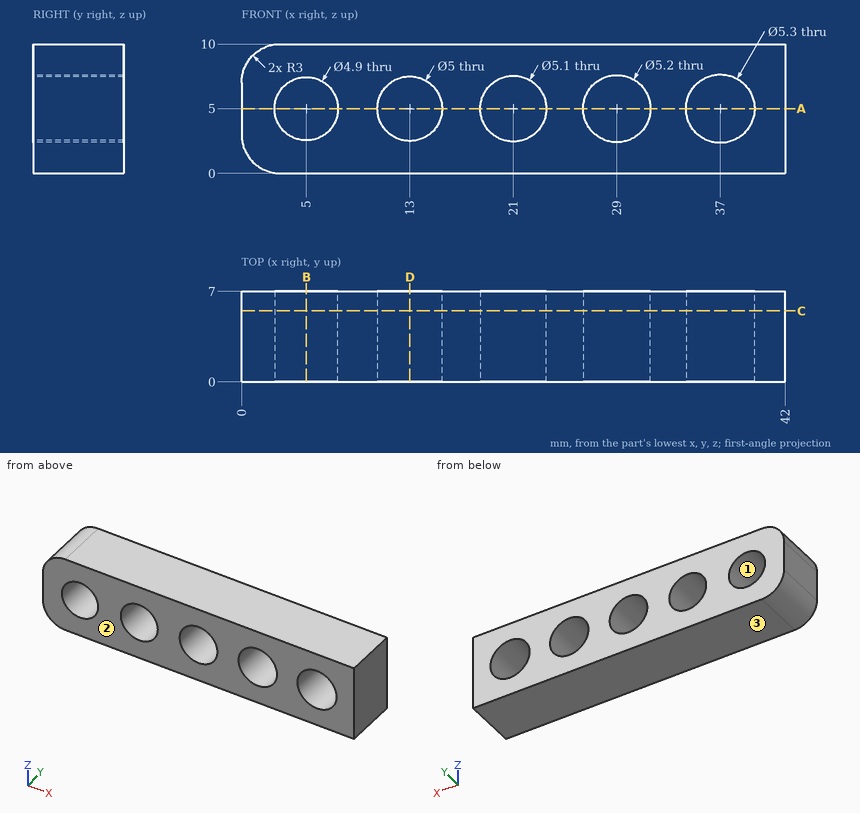
The figure shows three views and two pictorial views of one solid part (mm, origin at its lowest corner). Answer the questions. Round coordinates to 2 decimals unless told otherwise and drop trailing zeros. Order: outer loops, then holes, each group sorted by start corner. A loop starts at its lowest first (then second) coordinate and runs counter-clockwise, first axis right, second up. Notation, with made-up numbers: M 72,79.5 L 104,79.5 A18 ccw 104,88.5 Z; hole C 22,49 d11. An arc over 180 degrees is marked long. Put each result on its own line as item: value. Start each with the question number.
Q1. Section B-B, the plane x = 5 is taken. Write down the section's boundary in (y, z), and give its area (3 significant figures).
Q2. Section D-D, the plane x = 13 is taken. Write down the section's boundary in (y, z), and give its area (3 significant figures).
Q3. Section A-A, the plane z = 5 is taken. Write down the section's boundary in (x, y).
Q4. For a pull along Z with two mould halves and no side action, classify the marked faces 1, 2 and 3 as pulls with the +Z half, pulls with the -Z half, needs draft (parallel to the pull), parting line crosses it, or undercut.
Q5. Straight lines are drawn through the part: L1, parallel to X at y = 3, z = 5; L2, parallel to Z at x = 37.5, y = 2.25; L3, parallel to Z at x = 5, y = 1.75. For each, find the intervals that lie inside material, in ascending order. Write a range as [from, to].
Q6. Section C-C, the plane y = 5.5 is taken. Write down the section's boundary in (x, z), and give its area (3 significant figures).
Findings below:
1. outline: M 0,0 L 7,0 L 7,2.55 L 0,2.55 Z; M 0,7.45 L 7,7.45 L 7,10 L 0,10 Z
1. area: 35.7 mm^2
2. outline: M 0,0 L 7,0 L 7,2.5 L 0,2.5 Z; M 0,7.5 L 7,7.5 L 7,10 L 0,10 Z
2. area: 35.0 mm^2
3. outline: M 0,0 L 2.55,0 L 2.55,7 L 0,7 Z; M 7.45,0 L 10.5,0 L 10.5,7 L 7.45,7 Z; M 15.5,0 L 18.45,0 L 18.45,7 L 15.5,7 Z; M 23.55,0 L 26.4,0 L 26.4,7 L 23.55,7 Z; M 31.6,0 L 34.35,0 L 34.35,7 L 31.6,7 Z; M 39.65,0 L 42,0 L 42,7 L 39.65,7 Z
4. face 1: undercut
4. face 2: needs draft
4. face 3: pulls with the -Z half
5. L1: x = [0, 2.55], [7.45, 10.5], [15.5, 18.45], [23.55, 26.4], [31.6, 34.35], [39.65, 42]
5. L2: z = [0, 2.4], [7.6, 10]
5. L3: z = [0, 2.55], [7.45, 10]
6. outline: M 0,3 A3 ccw 3,0 L 42,0 L 42,10 L 3,10 A3 ccw 0,7 Z; hole C 5,5 d4.9; hole C 13,5 d5; hole C 21,5 d5.1; hole C 29,5 d5.2; hole C 37,5 d5.3
6. area: 314 mm^2
